Geometry check sheet. Reference: the model listing, model coordinates, mm. Face numbers are marked on the shaded views. A direction names the side the tool comes from. Round coordinates to 2 decimals unless told otherwise and drop trailing zeros. Loops run counter-clockwise (first coordinate to the right, second up) from the corner with the lowest first, then second, coordinate; pieces in that order, holes last. Notation, with made-up numbers: (73, 21.25) -> (86, 21.25) arc R28 cw to (86, 43.25) -> close; hole circle Ø2 at (3, -20). An arc over 180 degrees is marked (long way). Use one line per item in the form item = value.
from build123d import *

# Parameters (mm, degrees)
F0_R     = 49.654928
F1_DEPTH = 59.378261
F2_T     = -2.54
F3_W     = 100.591485
F3_H     = 104.532239
F4_DEPTH = 80.290629


with BuildPart() as f1:
    # F0 (on Top) → F1 (new body)
    with BuildSketch(Plane.XY):
        with Locations((0, -10.152236)):
            Circle(F0_R)
    extrude(amount=F1_DEPTH)

    # F2
    f2_openings = [f1.faces().sort_by_distance(p)[0] for p in [
        (0, -10.152236, 59.378261),
    ]]
    offset(amount=F2_T, openings=f2_openings)

    # F3 (on face) → F4 (join)
    with BuildSketch(Plane(origin=(0, 0, 0), x_dir=(1, 0, 0), z_dir=(0, 0, -1))):
        with Locations((-60.349798, 41.384102)):
            Rectangle(F3_W, F3_H)
    extrude(amount=-F4_DEPTH)


solid = f1.part
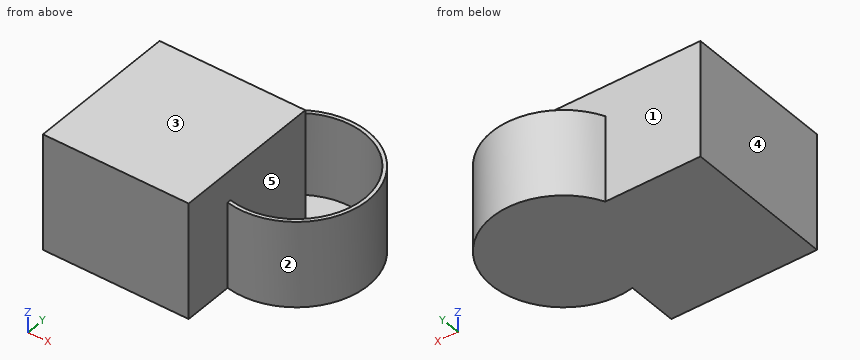
1. Tool access check on the marked faces 1 and 2. Record the directions out of +Z, -Z, +X, -X, +Y, -Y that give a thin tool (end or side, any length) a straight path to the whole face; none if there is none.
Return value:
face_1 = +Z
face_2 = +Z, -Z
2. Material ranges on line 1 along Y through (x, z) = (0, 20); line 2 along X through (y, z) = (-84, 61.5); line 3 along Y through (x, z) = (-94, 51), recorded low to high.
Return value:
line_1 = -59.81 to -57.27, 36.96 to 39.5
line_2 = -110.65 to -10.05
line_3 = -93.65 to 10.88
3. Section check A-A (x = 0). Record the boundary of the cut face in (y, z), then the cut area to 3 significant figures.
Return value:
outline = (-59.81, 0) -> (39.5, 0) -> (39.5, 59.38) -> (36.96, 59.38) -> (36.96, 2.54) -> (-57.27, 2.54) -> (-57.27, 59.38) -> (-59.81, 59.38) -> close
area = 541 mm2
4. Section check D-D (z = 72). Record the boundary of the cut face in (x, y), then the cut area to 3 significant figures.
Return value:
outline = (-110.65, -93.65) -> (-10.05, -93.65) -> (-10.05, 10.88) -> (-110.65, 10.88) -> close
area = 10,500 mm2
5. Gauge pin test, flat ends, axial feed: pin 1 (12 mm diameter, centred on y = -16.5, z = 33, fed in from +X); pin 2 (24 mm diameter, centred on x = -43.5, z = 55.5, fed in from +Y); pin 3 (12 mm diameter, centred on x = -59, z = 68.5, fed in from +Y). Record the tip position at first contact, or that the pin passes through.
Return value:
pin_1 = 49.65
pin_2 = 28.23
pin_3 = 10.88
6. Section check B-B (y = -14.5). Record the boundary of the cut face in (x, z), then the cut area to 3 significant figures.
Return value:
outline = (-110.65, 0) -> (49.46, 0) -> (49.46, 59.38) -> (46.91, 59.38) -> (46.91, 2.54) -> (-10.05, 2.54) -> (-10.05, 80.29) -> (-110.65, 80.29) -> close
area = 8,370 mm2
7. Mould release check, pull along X, two halves, no side actions. Record for the marked faces 3, 4 and 5: released by +X, released by -X, zero draft, split by the parting line, or undercut.
Return value:
face_3 = zero draft
face_4 = released by -X
face_5 = undercut
8. Section check C-C (z = 52). Record the boundary of the cut face in (x, y).
Return value:
outline = (-110.65, -93.65) -> (-10.05, -93.65) -> (-10.05, -58.78) arc R49.65 ccw (long way) to (-44.98, 10.88) -> (-110.65, 10.88) -> close; hole (-42.16, 10.88) -> (-10.05, 10.88) -> (-10.05, -56.18) arc R47.11 ccw (long way) to start
